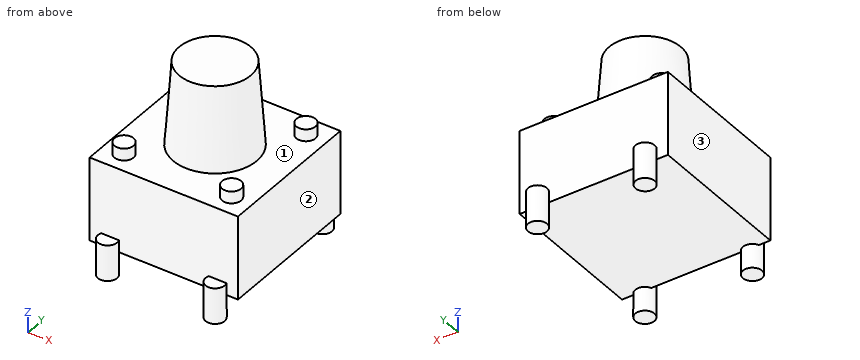
Autodesk Inventor part; units mm, degrees
ref_plane "YZ Plane" through (0, 0, 0) normal (1, 0, 0) x (0, 1, 0)
ref_plane "XZ Plane" through (0, 0, 0) normal (0, 1, 0) x (-1, 0, 0)
ref_plane "XY Plane" through (0, 0, 0) normal (0, 0, 1) x (1, 0, 0)
sketch "スケッチ1" plane through (0, 0, 0) normal (0, 0, 1) x (1, 0, 0)
  line L0 (-3.1, -3.1) -> (3.1, -3.1)
  line L1 (3.1, -3.1) -> (3.1, 3.1)
  line L2 (3.1, 3.1) -> (-3.1, 3.1)
  line L3 (-3.1, 3.1) -> (-3.1, -3.1)
  line L4 (-3.1, -3.1) -> (3.1, 3.1) construction
  line L5 (3.1, -3.1) -> (-3.1, 3.1) construction
  point P0 (0, 0)
  dimension "d0" = 6.2
  dimension "d2" = 6.2
extrude "押し出し1" add sketch "スケッチ1" along normal blind 3.5
sketch "スケッチ2" plane through (0, 0, 3.5) normal (0, 0, 1) x (1, 0, 0)
  line L0 (-2.25, -2.25) -> (2.25, -2.25) construction
  line L1 (2.25, -2.25) -> (2.25, 2.25) construction
  line L2 (2.25, 2.25) -> (-2.25, 2.25) construction
  line L3 (-2.25, 2.25) -> (-2.25, -2.25) construction
  line L4 (-2.25, -2.25) -> (2.25, 2.25) construction
  line L5 (2.25, -2.25) -> (-2.25, 2.25) construction
  circle A0 centre (-2.25, 2.25) radius 0.4
  circle A1 centre (2.25, 2.25) radius 0.4
  circle A2 centre (2.25, -2.25) radius 0.4
  circle A3 centre (-2.25, -2.25) radius 0.4
  point P0 (0, 0)
  dimension "d5" = 4.5
  dimension "d6" = 0.8
extrude "押し出し2" add sketch "スケッチ2" along normal blind 0.5
sketch "スケッチ3" plane through (0, 0, 0) normal (1, 0, 0) x (0, 1, 0)
  line L0 (3.1, 3.5) -> (-3.1, 3.5)
  line L1 (0, 3.5) -> (0, 7)
  line L2 (0, 7) -> (1.5, 7)
  line L3 (1.5, 7) -> (1.75, 3.5)
  line L4 (1.75, 3.5) -> (0, 3.5)
  point P0 (0, 0)
  dimension "d9" = 1.75
  dimension "d10" = 3.5
  dimension "d11" = 1.5
revolve "回転1" add sketch "スケッチ3" angle 360 about axis through (0, 0, 3.5) along (0, 0, 1)
sketch "スケッチ4" plane through (0, 0, 0) normal (0, 0, -1) x (-1, 0, 0)
  line L0 (2.25, -3.25) -> (-2.25, -3.25) construction
  line L1 (-2.25, -3.25) -> (-2.25, 3.25) construction
  line L2 (-2.25, 3.25) -> (2.25, 3.25) construction
  line L3 (2.25, 3.25) -> (2.25, -3.25) construction
  line L4 (2.25, -3.25) -> (-2.25, 3.25) construction
  line L5 (-2.25, -3.25) -> (2.25, 3.25) construction
  circle A0 centre (-2.25, 3.25) radius 0.4
  circle A1 centre (2.25, 3.25) radius 0.4
  circle A2 centre (2.25, -3.25) radius 0.4
  circle A3 centre (-2.25, -3.25) radius 0.4
  point P0 (0, 0)
  dimension "d13" = 4.5
  dimension "d14" = 6.5
  dimension "d15" = 0.8
extrude "押し出し3" add sketch "スケッチ4" along normal blind 1 and the other way blind 0.5
properties part number "DTS-6-V"
Here's how the part is built. I have some questions about the finished solid (model axes, mm). Face numbers are marked on the shaded views. Round coordinates to 2 decimals unless told otherwise and drop trailing zeros. Write each loop counter-clockwise with the first axis right and the second up, starting at its lowest first coordinate (ties: lowest second). Pieces come first, ordered by that corner, then holes.
Q1. Please list where these lines run through material, in increasing order: probe 1 along Z at (x, y) = (0, -0.25); probe 2 along Z at (x, y) = (3, -1.25); probe 3 along Y at (x, z) = (2.5, 1.5).
Q2. If we mould it in two halves opening along X, with no side actions, what happens to the marked faces 1, 2 and 3? For each: +X half, -X half, draft (parallel to the pull), parting line (faces both ways), or undercut.
Q3. If we section it at A-A on y = -3.25: Write out the boundary of the cut face in (x, z), plus the area to 3 significant figures.
Q4. If we section it at B-B on x = 2.25: Write out the boundary of the cut face in (y, z).
Q5. Will these pins go through, and if not, where does the flat tip stop? P1, Ø1, axis at x = -1, z = 1, coming from the -Y side; P2, Ø0.9, axis at x = -2, y = 2, coming from the +Z side; P3, Ø3, axis at x = 0.5, y = 1.5, coming from the -Z side; P4, Ø2, axis at x = 0.5, y = 2, coming from the +Z side.
Q6. If we section it at C-C on z = -0.5: Write out the boundary of the cut face in (x, y), plus the area to 3 significant figures.
Q7. If we section it at D-D on y = 0: Write out the boundary of the cut face in (x, z), plus the area to 3 significant figures.
Answer below:
1. probe 1: z = 0 to 7
1. probe 2: z = 0 to 3.5
1. probe 3: y = -3.1 to 3.1
2. face 1: undercut
2. face 2: +X half
2. face 3: -X half
3. outline: (-2.65, -1) - (-1.85, -1) - (-1.85, 0.5) - (-2.65, 0.5) - close; (1.85, -1) - (2.65, -1) - (2.65, 0.5) - (1.85, 0.5) - close
3. area: 2.40 mm2
4. outline: (-3.65, -1) - (-2.85, -1) - (-2.85, 0) - (2.85, 0) - (2.85, -1) - (3.65, -1) - (3.65, 0.5) - (3.1, 0.5) - (3.1, 3.5) - (2.65, 3.5) - (2.65, 4) - (1.85, 4) - (1.85, 3.5) - (-1.85, 3.5) - (-1.85, 4) - (-2.65, 4) - (-2.65, 3.5) - (-3.1, 3.5) - (-3.1, 0.5) - (-3.65, 0.5) - close
5. P1: stops at y = -3.1
5. P2: stops at z = 4
5. P3: stops at z = 0
5. P4: stops at z = 7
6. outline: circle Ø0.8 at (-2.25, -3.25); circle Ø0.8 at (-2.25, 3.25); circle Ø0.8 at (2.25, -3.25); circle Ø0.8 at (2.25, 3.25)
6. area: 2.01 mm2
7. outline: (-3.1, 0) - (3.1, 0) - (3.1, 3.5) - (1.75, 3.5) - (1.5, 7) - (-1.5, 7) - (-1.75, 3.5) - (-3.1, 3.5) - close
7. area: 33.1 mm2
